Geometry: final body of the model. Coordinates: model frame, mm. Face numbers are marked on the shaded views. A direction names the side the tool comes from. Coordinates: 2 decimals unless noted, no trailing zeros. Write each loop counter-clockwise with the first axis right and the second up, starting at its lowest first coordinate (ties: lowest second). Pieces come first, ordered by that corner, then holes.
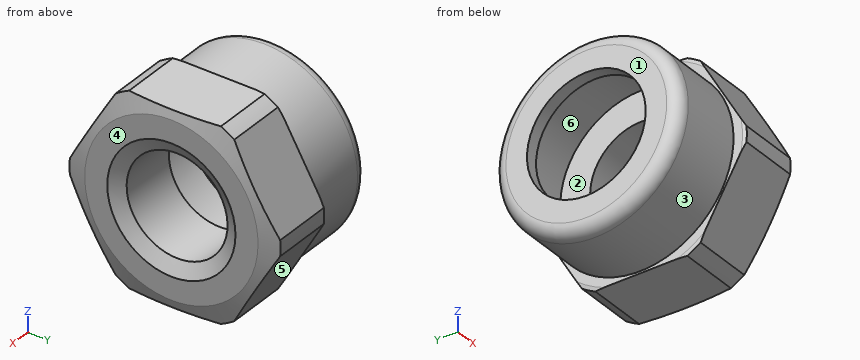
from build123d import *

# Parameters (mm, degrees)
SKETCH_2_OUTSIDE_W  = 25.332
SKETCH_2_OUTSIDE_H  = 25.332
CUT_EXTRUDE_1_DEPTH = 18.305965734


with BuildPart() as part:
    # Эскиз1 → Повернуть1 (revolve)
    with BuildSketch(Plane.XY, mode=Mode.PRIVATE) as revolve_1_sk:
        with BuildLine():
            Line((-11.9, 6.773556454), (-11.9, 5))
            Line((-11.9, 5), (-10.847112909, 5))
            Line((-10.847112909, 5), (-10.847112909, 6.773556454))
            Line((-10.847112909, 6.773556454), (-5.582677453, 6.773556454))
            Line((-5.582677453, 6.773556454), (-5.582677453, 4.25))
            Line((-5.582677453, 4.25), (0, 4.25))
            Line((0, 4.25), (0, 7.3))
            Line((0, 7.3), (-0.42469947, 8.885))
            Line((-0.42469947, 8.885), (-5.5, 8.885))
            Line((-5.5, 8.885), (-5.582677453, 8.576443546))
            Line((-5.582677453, 8.576443546), (-5.582677453, 7.826443546))
            Line((-5.582677453, 7.826443546), (-10.847112909, 7.826443546))
            ThreePointArc((-10.847112909, 7.826443546), (-11.591616511, 7.518060056), (-11.9, 6.773556454))
        make_face()
    revolve(revolve_1_sk.sketch.rotate(Axis((-1000, 0, 0), (1, 0, 0)), 90), axis=Axis((-1000, 0, 0), (1, 0, 0)))

    # Эскиз2 outside → Вырез-Вытянуть1 (cut, through all)
    with BuildSketch(Plane(origin=(0, 0, 0), x_dir=(0, 0, -1), z_dir=(1, 0, 0))):
        Rectangle(SKETCH_2_OUTSIDE_W, SKETCH_2_OUTSIDE_H)
        Polygon((8, -4.618802154), (8, 4.618802154), (0, 9.237604307), (-8, 4.618802154), (-8, -4.618802154), (0, -9.237604307), align=None, mode=Mode.SUBTRACT)
    extrude(amount=-CUT_EXTRUDE_1_DEPTH, mode=Mode.SUBTRACT)

    # Эскиз3 → Вырез-Повернуть1 (revolve, cut)
    with BuildSketch(Plane.XY, mode=Mode.PRIVATE) as cut_revolve_1_sk:
        Polygon((0, 0), (0, 5.4), (-0.66395281, 4.25), (-0.66395281, 0), align=None)
    revolve(cut_revolve_1_sk.sketch.rotate(Axis((-0.66395281, 0, 0), (1.0, -1.853694946210833e-11, 0)), 90.000000001), axis=Axis((-0.66395281, 0, 0), (1.0, -1.853694946210833e-11, 0)), mode=Mode.SUBTRACT)


solid = part.part
Item 1: Set-up query: the marked faces 1, 2 and 3. Return all of +Z, -Z, +X, -X, +Y, -Y with unobstructed straight access to the full face (end or side cutting, diameter ignored); none if empty.
Derived:
face 1: +Z, -Z, -X, +Y, -Y
face 2: none
face 3: -X
Item 2: Pull-direction query (Z, two-part tool) for the marked faces 4, 5 and 6; classes: released by +Z, released by -Z, zero draft, split by the parting line, or undercut.
Derived:
face 4: zero draft
face 5: released by -Z
face 6: undercut
Item 3: Section C-C, the plane x = -5.25. Output: boundary loops of the cut face in (y, z) (3 decimals).
Derived:
outline: (-8.861, -0.652) - (-4.995, -7.348) arc R8.885 ccw to (-3.866, -8) - (3.866, -8) arc R8.885 ccw to (4.995, -7.348) - (8.861, -0.652) arc R8.885 ccw to (8.861, 0.652) - (4.995, 7.348) arc R8.885 ccw to (3.866, 8) - (-3.866, 8) arc R8.885 ccw to (-4.995, 7.348) - (-8.861, 0.652) arc R8.885 ccw to start; hole circle Ø8.5 at (0, 0)
Item 4: Pin query (flat end, axial travel): pin 1 (3 mm diameter, centred on x = -10.5, z = 4.5, fed in from -Y); pin 2 (8 mm diameter, centred on y = 0.5, z = 0.5, fed in from -X); pin 3 (1 mm diameter, centred on x = -8.5, z = -4, fed in from +Y). Return the tip coordinate at first contact, or that it passes through.
Derived:
pin 1: stops at y = -7.23
pin 2: stops at x = -5.58
pin 3: stops at y = 7
Item 5: Material intervals for probe 1 along Y at (x, z) = (-8.3, 0); probe 2 along X at (y, z) = (-6.5, -0.5); probe 3 along Z at (x, y) = (-1.5, 0), sorted ascending.
Derived:
probe 1: y = -7.83 to -6.77, 6.77 to 7.83
probe 2: x = -11.9 to -10.85, -5.58 to 0
probe 3: z = -8 to -4.25, 4.25 to 8
Item 6: Section A-A, the plane y = 0. Output: boundary loops of the cut face in (x, z), plus the area to 3 significant figures.
Derived:
outline: (-11.9, -6.77) arc R1.05 ccw to (-10.85, -7.83) - (-5.58, -7.83) - (-5.58, -8) - (-0.19, -8) - (0, -7.3) - (0, -5.4) - (-0.66, -4.25) - (-5.58, -4.25) - (-5.58, -6.77) - (-10.85, -6.77) - (-10.85, -5) - (-11.9, -5) - close; (-11.9, 5) - (-10.85, 5) - (-10.85, 6.77) - (-5.58, 6.77) - (-5.58, 4.25) - (-0.66, 4.25) - (0, 5.4) - (0, 7.3) - (-0.19, 8) - (-5.58, 8) - (-5.58, 7.83) - (-10.85, 7.83) arc R1.05 ccw to (-11.9, 6.77) - close
area: 57.5 mm2
Item 7: Section B-B, the plane z = 0. Output: boundary loops of the cut face in (x, y) (3 decimals).
Derived:
outline: (-11.9, -6.774) arc R1.053 ccw to (-10.847, -7.826) - (-5.583, -7.826) - (-5.583, -8.576) - (-5.5, -8.885) - (-0.425, -8.885) - (0, -7.3) - (0, -5.4) - (-0.664, -4.25) - (-5.583, -4.25) - (-5.583, -6.774) - (-10.847, -6.774) - (-10.847, -5) - (-11.9, -5) - close; (-11.9, 5) - (-10.847, 5) - (-10.847, 6.774) - (-5.583, 6.774) - (-5.583, 4.25) - (-0.664, 4.25) - (0, 5.4) - (0, 7.3) - (-0.425, 8.885) - (-5.5, 8.885) - (-5.583, 8.576) - (-5.583, 7.826) - (-10.847, 7.826) arc R1.053 ccw to (-11.9, 6.774) - close
Item 8: Section D-D, the plane x = -7.25. Output: boundary loops of the cut face in (y, z), plus the area to 3 significant figures.
Derived:
outline: circle Ø15.65 at (0, 0); hole circle Ø13.55 at (0, 0)
area: 48.3 mm2
